CAD build for the part. Positions are in the model's coordinates, mm. Face numbers are marked on the shaded views. A direction names the side the tool comes from. Round coordinates to 2 decimals unless told otherwise and drop trailing zeros. Write each loop counter-clockwise with the first axis right and the second up, starting at its lowest first coordinate (ties: lowest second). Pieces come first, ordered by that corner, then holes. Notation, with made-up numbers: (21.5, 64.25) - (50.5, 64.25) arc R11 cw to (50.5, 81.25) - close; hole circle Ø1 at (36.5, -10.5). An arc over 180 degrees is marked (long way). Use one line per item in the form item = value. Start each with the question number.
Item 1: Band-saw the part on D-D, the plane y = 21.5. Give the number of separate pieces and of enclosed holes in the cut face, and give its area (3 significant figures).
Item 2: Tool access for the marked faces 1, 2, 3 and 4: list every direction of +Z, -Z, +X, -X, +Y, -Y with a clear straight run to the whole face (end or side of a thin tool).
Item 3: Band-saw the part on A-A, the plane x = 0. List the corners of the cut face in (y, z), and give its area (3 significant figures).
Item 4: Band-saw the part on B-B, the plane z = 29.75. List the corners of the cut face in (x, y) (3 decimals).
Item 5: Drill centre lines: L1, parallel to X at y = -2.8, z = 0; L2, parallel to X at y = 10, z = 19.5. Where is each one in solid material? Low to high.
Item 6: Pull direction X, two halves, no side cores. Call the marked faces 5, 6 and 7: +X half, -X half, draft (parallel to the pull), parting line (faces both ways), or undercut.
Item 7: Pin check, flat tips, straight feed: pin 1 (10 mm diameter, centred on x = 0, z = 29.75, fed in from -Y); pin 2 (1.1 mm diameter, centred on y = 9, z = 18, fed in from -X); pin 3 (1.3 mm diameter, centred on y = 25.5, z = 22.5, fed in from -X); pin 4 (9.5 mm diameter, centred on x = 2, z = 32, fed in from +Y). Stop position of each tip, or through.
Item 8: Band-saw the part on C-C, the plane x = -29.75. List the corners of the cut face in (y, z) (3 decimals).
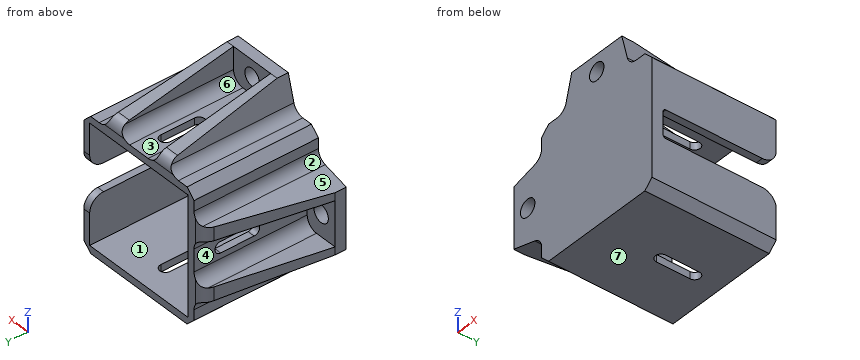
from build123d import *

# Parameters (mm, degrees)
SKETCH1_W                = 47.5
SKETCH1_H                = 47.5
SKETCH1_W_2              = 42.4
SKETCH1_H_2              = 42.4
BOSS_EXTRUDE1_DEPTH      = 40.5
FILLET1_SIZE             = 3
BOSS_EXTRUDE3_DEPTH      = 10
BOSS_EXTRUDE3_DEPTH_BACK = 10
CUT_EXTRUDE1_DEPTH       = 8
CUT_EXTRUDE1_DEPTH_BACK  = 8
BOSS_EXTRUDE4_DEPTH      = 10
BOSS_EXTRUDE4_DEPTH_BACK = 10
CUT_EXTRUDE2_DEPTH       = 8
CUT_EXTRUDE2_DEPTH_BACK  = 8
BOSS_EXTRUDE6_DEPTH      = 4
SKETCH10_R               = 3.1
CUT_EXTRUDE3_DEPTH       = 65.779433465
SKETCH11_R               = 3.1
CUT_EXTRUDE4_DEPTH       = 65.779433465
SKETCH14_W               = 5
SKETCH14_H               = 40.5
CUT_EXTRUDE6_DEPTH       = 10
FILLET9_R                = 5
FILLET10_R               = 1
CUT_EXTRUDE7_DEPTH       = 2.55
CUT_EXTRUDE8_DEPTH       = 72.93443195
CHAMFER1_SIZE            = 4
CHAMFER1_SIZE_2          = 14.92820323
CHAMFER2_SIZE            = 4
CHAMFER2_SIZE_2          = 14.92820323
CHAMFER3_SIZE            = 4
CHAMFER3_SIZE_2          = 14.92820323
FILLET16_R               = 4
FILLET17_R               = 4


with BuildPart() as part:
    # Sketch1 → Boss-Extrude1 (new body)
    with BuildSketch(Plane(origin=(0, 0, 0), x_dir=(1, 0, 0), z_dir=(0, 1, 0))):
        Rectangle(SKETCH1_W, SKETCH1_H)
        Rectangle(SKETCH1_W_2, SKETCH1_H_2, mode=Mode.SUBTRACT)
    extrude(amount=BOSS_EXTRUDE1_DEPTH)

    # Fillet1
    fillet1_edges = [part.edges().sort_by_distance(p)[0] for p in [
        (23.75, 20.25, 23.75),
        (-23.75, 20.25, 23.75),
        (-23.75, 20.25, -23.75),
        (23.75, 20.25, -23.75),
    ]]
    chamfer(fillet1_edges, length=FILLET1_SIZE)

    # Sketch3 → Boss-Extrude3 (add, two sides: drawn at the far end of the back side and taken through both)
    with BuildSketch(Plane.XY.offset(-BOSS_EXTRUDE3_DEPTH_BACK)):
        Polygon((-23.75, 0), (-23.75, 40.5), (-27.75, 40.5), (-35.75, 0), align=None)
    extrude(amount=BOSS_EXTRUDE3_DEPTH + BOSS_EXTRUDE3_DEPTH_BACK)

    # Sketch4 → Cut-Extrude1 (cut, two sides: drawn at the far end of the back side and taken through both)
    with BuildSketch(Plane.XY.offset(-CUT_EXTRUDE1_DEPTH_BACK)):
        Polygon((-35.75, 0), (-23.75, 0), (-23.75, 40.5), (-27.75, 40.5), align=None)
    extrude(amount=CUT_EXTRUDE1_DEPTH + CUT_EXTRUDE1_DEPTH_BACK, mode=Mode.SUBTRACT)

    # Sketch7 → Boss-Extrude4 (add, two sides: drawn at the far end of the back side and taken through both)
    with BuildSketch(Plane(origin=(0, 0, 0), x_dir=(0, 0, -1), z_dir=(1, 0, 0)).offset(-BOSS_EXTRUDE4_DEPTH_BACK)):
        Polygon((-35.75, 0), (-23.75, 0), (-23.75, 40.5), (-27.75, 40.5), align=None)
    extrude(amount=BOSS_EXTRUDE4_DEPTH + BOSS_EXTRUDE4_DEPTH_BACK)

    # Sketch8 → Cut-Extrude2 (cut, two sides: drawn at the far end of the back side and taken through both)
    with BuildSketch(Plane(origin=(0, 0, 0), x_dir=(0, 0, -1), z_dir=(1, 0, 0)).offset(-CUT_EXTRUDE2_DEPTH_BACK)):
        Polygon((-23.75, 0), (-23.75, 40.5), (-27.75, 40.5), (-35.75, 0), align=None)
    extrude(amount=CUT_EXTRUDE2_DEPTH + CUT_EXTRUDE2_DEPTH_BACK, mode=Mode.SUBTRACT)

    # Sketch9 → Boss-Extrude6 (add)
    with BuildSketch(Plane(origin=(0, 0, 0), x_dir=(1, 0, 0), z_dir=(0, 1, 0))):
        Polygon((-35.75, -10), (-23.75, -10), (-23.75, -20.75), (-20.75, -23.75), (-10, -23.75), (-10, -35.75), (10, -35.75), (10, -23.75), (20.75, -23.75), (23.75, -20.75), (23.75, 20.75), (20.75, 23.75), (-20.75, 23.75), (-23.75, 20.75), (-23.75, 10), (-35.75, 10), align=None)
    extrude(amount=-BOSS_EXTRUDE6_DEPTH)

    # Sketch10 → Cut-Extrude3 (cut, through all)
    with BuildSketch(Plane(origin=(0, 0, 0), x_dir=(1, 0, 0), z_dir=(0, 1, 0))):
        with Locations(Location((-29.75, 0, 0), (0, 0, 270))):
            Circle(SKETCH10_R)
    extrude(amount=-CUT_EXTRUDE3_DEPTH, mode=Mode.SUBTRACT)

    # Sketch11 → Cut-Extrude4 (cut, through all)
    with BuildSketch(Plane(origin=(0, 0, 0), x_dir=(1, 0, 0), z_dir=(0, 1, 0))):
        with Locations(Location((0, -29.75, 0), (0, 0, 270))):
            Circle(SKETCH11_R)
    extrude(amount=-CUT_EXTRUDE4_DEPTH, mode=Mode.SUBTRACT)

    # Sketch14 → Cut-Extrude6 (cut)
    with BuildSketch(Plane(origin=(23.75, 0, 0), x_dir=(0, 0, -1), z_dir=(1, 0, 0))):
        with Locations((-2.5, 20.25)):
            Rectangle(SKETCH14_W, SKETCH14_H)
        with Locations((2.5, 20.25)):
            Rectangle(SKETCH14_W, SKETCH14_H)
    extrude(amount=-CUT_EXTRUDE6_DEPTH, mode=Mode.SUBTRACT)

    # Fillet9
    fillet9_edges = [part.edges().sort_by_distance(p)[0] for p in [
        (22.475, 40.5, 5),
        (22.475, 40.5, -5),
    ]]
    fillet(fillet9_edges, radius=FILLET9_R)

    # Fillet10
    fillet10_edges = [part.edges().sort_by_distance(p)[0] for p in [
        (22.475, 0, -5),
        (22.475, 0, 5),
    ]]
    fillet(fillet10_edges, radius=FILLET10_R)

    # Sketch15 → Cut-Extrude7 (cut)
    with BuildSketch(Plane.ZY.offset(23.75)):
        with BuildLine():
            Line((-2, 19), (-2, 31))
            ThreePointArc((-2, 31), (0, 33), (2, 31))
            Line((2, 31), (2, 19))
            ThreePointArc((2, 19), (0, 17), (-2, 19))
        make_face()
    extrude(amount=-CUT_EXTRUDE7_DEPTH, mode=Mode.SUBTRACT)

    # Sketch16 → Cut-Extrude8 (cut, through all)
    with BuildSketch(Plane.XY.offset(23.75)):
        with BuildLine():
            Line((2, 31), (2, 19))
            ThreePointArc((2, 19), (0, 17), (-2, 19))
            Line((-2, 19), (-2, 31))
            ThreePointArc((-2, 31), (0, 33), (2, 31))
        make_face()
    extrude(amount=-CUT_EXTRUDE8_DEPTH, mode=Mode.SUBTRACT)

    # Chamfer1
    # the kernel refuses this chamfer: 14.92820323, 4 mm, written as the material it adds along each edge
    with BuildSketch(Plane(origin=(10, 40.5, 23.75), x_dir=(0.9905000388259542, 0, -0.13751244702129095), z_dir=(0, -1, 0))) as chamfer1_piece_1_section:
        Polygon((CHAMFER1_SIZE * 0.990500038826, CHAMFER1_SIZE * 0.137512447021), (-CHAMFER1_SIZE_2 * 0.137512447024, CHAMFER1_SIZE_2 * 0.990500038844), (0, 0), align=None)
    chamfer1_piece_1 = extrude(amount=44.5, mode=Mode.PRIVATE)
    chamfer1_piece_1 = split(chamfer1_piece_1, bisect_by=Plane(origin=(11.413878062, 16.831768276, 32.425206267), z_dir=(0, -0.19378641821299017, -0.9810437422032618)), keep=Keep.TOP, mode=Mode.PRIVATE)
    chamfer1_piece_1 = split(chamfer1_piece_1, bisect_by=Plane(origin=(11.413878062, 15.820324331, 35.75), z_dir=(0, 0, -1)), keep=Keep.TOP, mode=Mode.PRIVATE)
    add(chamfer1_piece_1)
    with BuildSketch(Plane(origin=(-23.75, 40.5, 10), x_dir=(-0.9999503267608394, 0, -0.009967146577156315), z_dir=(0, -1, 0))) as chamfer1_piece_2_section:
        Polygon((CHAMFER1_SIZE_2 * 0.999950326779, -CHAMFER1_SIZE_2 * 0.00996714657734), (-CHAMFER1_SIZE * 0.00996714657716, -CHAMFER1_SIZE * 0.999950326761), (0, 0), align=None)
    chamfer1_piece_2 = extrude(amount=44.5, mode=Mode.PRIVATE)
    chamfer1_piece_2 = split(chamfer1_piece_2, bisect_by=Plane(origin=(-32.425206267, 16.831768276, 11.413878062), z_dir=(0.9810437422032618, -0.19378641821299017, 0)), keep=Keep.TOP, mode=Mode.PRIVATE)
    chamfer1_piece_2 = split(chamfer1_piece_2, bisect_by=Plane(origin=(-35.75, 15.820324331, 11.413878062), z_dir=(1, 0, 0)), keep=Keep.TOP, mode=Mode.PRIVATE)
    add(chamfer1_piece_2)

    # Chamfer2
    # the kernel refuses this chamfer: 14.92820323, 4 mm, written as the material it adds along each edge
    with BuildSketch(Plane(origin=(-23.75, 40.5, -10), x_dir=(0.13751244702129095, 0, -0.9905000388259542), z_dir=(0, -1, 0))) as chamfer2_piece_1_section:
        Polygon((CHAMFER2_SIZE * 0.990500038826, -CHAMFER2_SIZE * 0.137512447021), (-CHAMFER2_SIZE_2 * 0.137512447024, -CHAMFER2_SIZE_2 * 0.990500038844), (0, 0), align=None)
    chamfer2_piece_1 = extrude(amount=44.5, mode=Mode.PRIVATE)
    chamfer2_piece_1 = split(chamfer2_piece_1, bisect_by=Plane(origin=(-32.425206267, 16.831768276, -11.413878062), z_dir=(0.9810437422032618, -0.19378641821299017, 0)), keep=Keep.TOP, mode=Mode.PRIVATE)
    chamfer2_piece_1 = split(chamfer2_piece_1, bisect_by=Plane(origin=(-35.75, 15.820324331, -11.413878062), z_dir=(1, 0, 0)), keep=Keep.TOP, mode=Mode.PRIVATE)
    add(chamfer2_piece_1)

    # Chamfer3
    # the kernel refuses this chamfer: 14.92820323, 4 mm, written as the material it adds along each edge
    with BuildSketch(Plane(origin=(-10, -4, 23.75), x_dir=(-0.9905000388259542, 0, -0.13751244702129095), z_dir=(0, 1, 0))) as chamfer3_piece_1_section:
        Polygon((CHAMFER3_SIZE * 0.990500038826, CHAMFER3_SIZE * 0.137512447021), (-CHAMFER3_SIZE_2 * 0.137512447024, CHAMFER3_SIZE_2 * 0.990500038844), (0, 0), align=None)
    chamfer3_piece_1 = extrude(amount=44.5, mode=Mode.PRIVATE)
    chamfer3_piece_1 = split(chamfer3_piece_1, bisect_by=Plane(origin=(-11.413878062, 16.831768276, 32.425206267), z_dir=(0, -0.19378641821299017, -0.9810437422032618)), keep=Keep.TOP, mode=Mode.PRIVATE)
    chamfer3_piece_1 = split(chamfer3_piece_1, bisect_by=Plane(origin=(-11.413878062, 15.820324331, 35.75), z_dir=(0, 0, -1)), keep=Keep.TOP, mode=Mode.PRIVATE)
    add(chamfer3_piece_1)

    # Fillet16
    fillet16_edges = [part.edges().sort_by_distance(p)[0] for p in [
        (-8, 20.25, 23.75),
        (8, 20.25, 23.75),
        (-23.75, 18.25, 14),
        (14, 18.25, 23.75),
        (-23.75, 18.25, -14),
        (-14, 18.25, 23.75),
        (-23.75, 20.25, -8),
        (-23.75, 20.25, 8),
    ]]
    fillet(fillet16_edges, radius=FILLET16_R)

    # Fillet17
    fillet17_edges = [part.edges().sort_by_distance(p)[0] for p in [
        (-27.75, 40.5, -10.464101615),
        (-27.75, 40.5, 10.464101615),
        (-10.464101615, 40.5, 27.75),
        (10.464101615, 40.5, 27.75),
    ]]
    fillet(fillet17_edges, radius=FILLET17_R)


solid = part.part
Determined:
q1.separate_pieces = 4
q1.enclosed_holes = 0
q1.area = 559 mm²
q2.face_1 = +Y
q2.face_2 = +Z, -X, +Y, -Y
q2.face_3 = +Z, +Y
q2.face_4 = -X, +Y
q3.outline = (-4, -23.75) - (17, -23.75) - (17, -21.2) - (0, -21.2) - (0, 21.2) - (17, 21.2) - (17, 23.75) - (0, 23.75) - (0, 26.65) - (-4, 26.65) - close; (-4, 32.85) - (0, 32.85) - (0, 35.75) - (-4, 35.75) - close; (33, -23.75) - (40.5, -23.75) - (40.5, -21.2) - (33, -21.2) - close; (33, 21.2) - (40.5, 21.2) - (40.5, 23.75) - (33, 23.75) - close
q3.area = 338 mm²
q4.outline = (-12.392, -4) - (-3.1, -4) - (-3.1, 0) - (-8, 0) - (-8, 30.375) - (-12.392, 30.375) - close; (3.1, -4) - (12.392, -4) - (12.392, 30.375) - (8, 30.375) - (8, 0) - (3.1, 0) - close
q5.L1 = -35.75 to -32.85, -26.65 to 23.75
q5.L2 = -23.75 to -21.2, 21.2 to 23.75
q6.face_5 = -X half
q6.face_6 = undercut
q6.face_7 = draft
q7.pin_1 = -4
q7.pin_2 = -23.75
q7.pin_3 = -22.65
q7.pin_4 = 0
q8.outline = (-4, -12.392) - (30.375, -12.392) - (30.375, -8) - (0, -8) - (0, -3.1) - (-4, -3.1) - close; (-4, 3.1) - (0, 3.1) - (0, 8) - (30.375, 8) - (30.375, 12.392) - (-4, 12.392) - close
